Work out the finished part from the listing and answer in its coordinate system (mm). A direction names the side the tool comes from. Give positions to 0.01 mm unless a question says otherwise; leave off trailing zeros. Order: outer loops, then holes, each group sorted by start corner. A loop starts at its lowest first (then second) coordinate and runs counter-clockwise, first axis right, second up. Notation, with made-up numbers: (57.5, -34) - (105.5, -34) arc R22 ccw to (105.5, -1) - close; hole circle Ø4 at (52.25, 4). An arc over 180 degrees is marked (long way). Write each question's results on one line, items separated by ' | '.
from build123d import *

# Parameters (mm, degrees)
ESQUISSE2_W                  = 4.45
ESQUISSE2_H                  = 5.6
ESQUISSE3_R                  = 10.45
ESQUISSE3_R_2                = 0.75
BOSS_EXTRU_1_DEPTH           = 2.3
ESQUISSE4_R                  = 2.95
ENL_V_MAT_EXTRU_1_DEPTH      = 1.05
ESQUISSE5_R                  = 4.65
ESQUISSE5_R_2                = 3.35
ENL_V_MAT_EXTRU_2_DEPTH      = 1.05
ESQUISSE6_R                  = 1.5
ENL_V_MAT_EXTRU_3_DEPTH      = 6.6
ESQUISSE8_R                  = 2.68
ENL_V_MAT_EXTRU_4_DEPTH      = 4.5
ENL_V_MAT_EXTRU_5_DEPTH      = 4.5
R_P_TITION_CIRCULAIRE1_COUNT = 25


with BuildPart() as part:
    # Esquisse2 → Révolution1 (revolve)
    with BuildSketch(Plane.XY):
        with Locations((-2.225, -0.7)):
            Rectangle(ESQUISSE2_W, ESQUISSE2_H)
    revolve(axis=Axis((0, 3.929571688, 0), (0, -1, 0)))

    # Esquisse3 → Boss.-Extru.1 (add)
    with BuildSketch(Plane(origin=(0, 2.1, 0), x_dir=(1, 0, 0), z_dir=(0, 1, 0))):
        Circle(ESQUISSE3_R)
        with Locations((-3.4, 7.071067812)):
            Circle(ESQUISSE3_R_2, mode=Mode.SUBTRACT)
        with Locations((0, 7.071067812)):
            Circle(ESQUISSE3_R_2, mode=Mode.SUBTRACT)
        with Locations((3.4, 7.071067812)):
            Circle(ESQUISSE3_R_2, mode=Mode.SUBTRACT)
        with Locations((-7.071067812, 3.4)):
            Circle(ESQUISSE3_R_2, mode=Mode.SUBTRACT)
        with Locations((-7.071067812, 0)):
            Circle(ESQUISSE3_R_2, mode=Mode.SUBTRACT)
        with Locations((-7.071067812, -3.4)):
            Circle(ESQUISSE3_R_2, mode=Mode.SUBTRACT)
        with Locations((-3.4, -7.071067812)):
            Circle(ESQUISSE3_R_2, mode=Mode.SUBTRACT)
        with Locations((0, -7.071067812)):
            Circle(ESQUISSE3_R_2, mode=Mode.SUBTRACT)
        with Locations((3.4, -7.071067812)):
            Circle(ESQUISSE3_R_2, mode=Mode.SUBTRACT)
        with Locations((7.071067812, 3.4)):
            Circle(ESQUISSE3_R_2, mode=Mode.SUBTRACT)
        with Locations((7.071067812, 0)):
            Circle(ESQUISSE3_R_2, mode=Mode.SUBTRACT)
        with Locations((7.071067812, -3.4)):
            Circle(ESQUISSE3_R_2, mode=Mode.SUBTRACT)
    extrude(amount=-BOSS_EXTRU_1_DEPTH)

    # Esquisse4 → Enlèv. mat.-Extru.1 (cut)
    with BuildSketch(Plane(origin=(0, 2.1, 0), x_dir=(1, 0, 0), z_dir=(0, 1, 0))):
        Circle(ESQUISSE4_R)
    extrude(amount=-ENL_V_MAT_EXTRU_1_DEPTH, mode=Mode.SUBTRACT)

    # Esquisse5 → Enlèv. mat.-Extru.2 (cut)
    with BuildSketch(Plane(origin=(0, 2.1, 0), x_dir=(1, 0, 0), z_dir=(0, 1, 0))):
        Circle(ESQUISSE5_R)
        Circle(ESQUISSE5_R_2, mode=Mode.SUBTRACT)
    extrude(amount=-ENL_V_MAT_EXTRU_2_DEPTH, mode=Mode.SUBTRACT)

    # Esquisse6 → Enlèv. mat.-Extru.3 (cut, through all)
    with BuildSketch(Plane.XZ.offset(3.5)):
        Circle(ESQUISSE6_R)
    extrude(amount=-ENL_V_MAT_EXTRU_3_DEPTH, mode=Mode.SUBTRACT)

    # Esquisse8 → Enlèv. mat.-Extru.4 (cut, through all)
    with BuildSketch(Plane(origin=(0, 0, 0), x_dir=(1, 0, 0), z_dir=(0, 1, 0))):
        Circle(ESQUISSE8_R)
    extrude(amount=-ENL_V_MAT_EXTRU_4_DEPTH, mode=Mode.SUBTRACT)

    # Esquisse9 → Enlèv. mat.-Extru.5 (cut, through all)
    with BuildSketch(Plane(origin=(0, 0, 0), x_dir=(1, 0, 0), z_dir=(0, 1, 0))):
        with BuildLine():
            Line((0.10528472, -3.048182266), (0.265600366, -2.666806413))
            ThreePointArc((0.265600366, -2.666806413), (0, -2.68), (-0.265600366, -2.666806413))
            Line((-0.265600366, -2.666806413), (-0.10528472, -3.048182266))
            ThreePointArc((-0.10528472, -3.048182266), (0, -3.05), (0.10528472, -3.048182266))
        make_face()
    enl_v_mat_extru_5 = extrude(amount=-ENL_V_MAT_EXTRU_5_DEPTH, mode=Mode.SUBTRACT)

    # Répétition circulaire1: Enlèv. mat.-Extru.5 ×25 about axis
    r_p_tition_circulaire1_axis = Axis((0, 0, 0), (0, 1, 0))
    for i in range(1, R_P_TITION_CIRCULAIRE1_COUNT):
        add(enl_v_mat_extru_5.rotate(r_p_tition_circulaire1_axis, i * 360 / R_P_TITION_CIRCULAIRE1_COUNT), mode=Mode.SUBTRACT)


solid = part.part
1. Given P1, Ø1.8, axis at x = 0, z = 0, coming from the +Y side; P2, Ø1.7, axis at x = 0, z = -7.07, coming from the -Y side; P3, Ø1, axis at x = 1, y = 1, coming from the -Z side; P4, Ø1.5, axis at x = -3.5, y = -2, coming from the +Z side, each flat-ended and moving along its own axis, determine where each tip first touches the part or whether it passes through.
Answer list:
P1: through | P2: y = -0.2 | P3: z = -10.44 | P4: z = 3.5
2. A tool of negligible diameter and unlimited length cuts with its end or side. For faces 1 (the face through (1.3, 1.05, 1.3)), 2 (the face through (6.908, 0.966, 4.132)), 3 (the face through (4.5, -0.2, 2.2)), from which of +Z, -Z, +X, -X, +Y, -Y can it reach the whole face along a straight path? Write none if from no direction.
Answer list:
face 1: +Y | face 2: +Y, -Y | face 3: -Y
3. A cutting plane is placed at A-A, the plane x = 5.75. Write down the section's boundary in (y, z), then the cut area to 3 significant figures.
Answer list:
outline: (-0.2, -8.73) - (2.1, -8.73) - (2.1, 8.73) - (-0.2, 8.73) - close | area: 40.1 mm^2
4. Determine the mould class of faces 4 (the face through (0.965, -1.827, 4.344)), 5 (the face through (0, -3.5, -3)), 6 (the face through (-0.16, 0.97, -6.34)), 7 (the face through (3, 1.05, 2)) for opening direction Z: +Z half, -Z half, draft (parallel to the pull), parting line (faces both ways), or undercut.
Answer list:
face 4: parting line | face 5: draft | face 6: undercut | face 7: undercut
5. Straight lines are drawn through the part: line 1 (Z direction, x = 0, y = 1.3); line 2 (Z direction, x = -3.4, y = 0.3); line 3 (Y direction, x = -0.5, z = 2). For each, find the intervals that lie inside material, in ascending order. Write a range as [from, to].
Answer list:
line 1: [-10.45, -7.82], [-6.32, -4.65], [-3.35, -2.95], [2.95, 3.35], [4.65, 6.32], [7.82, 10.45] | line 2: [-9.88, -7.82], [-6.32, 6.32], [7.82, 9.88] | line 3: [0, 1.05]
